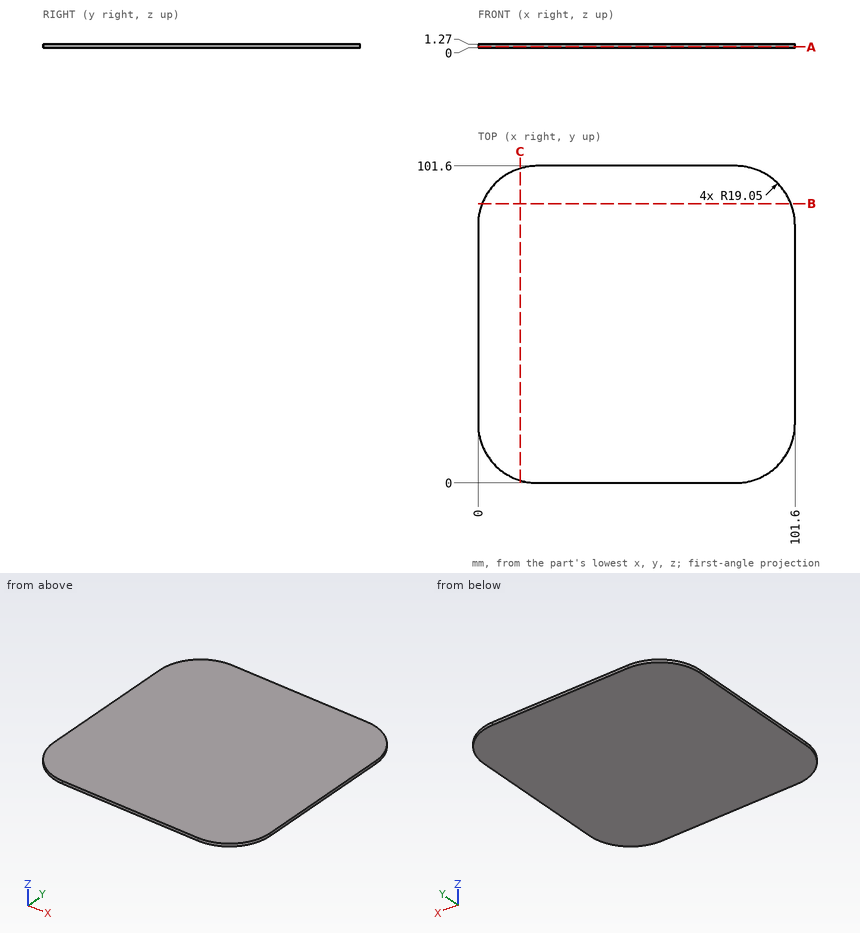
Part print with two shaded views. Sizes in mm from the minimum x, y, z corner. Round coordinates to 2 decimals unless told otherwise and drop trailing zeros. Loops run counter-clockwise (first coordinate to the right, second up) from the corner with the lowest first, then second, coordinate; pieces in that order, holes last. Notation, with made-up numbers: (26, 58) - (40, 58) arc R26 ccw to (40, 97) - close; hole circle Ø1 at (11.25, 32). An arc over 180 degrees is marked (long way). Put each result on its own line as item: value.
1. Slice it at B-B on y = 89.5. List the corners of the cut face in (x, z).
Geometry check:
outline: (1.31, 0) - (100.29, 0) - (100.29, 1.27) - (1.31, 1.27) - close
2. Slice it at A-A on z = 0.35. List the corners of the cut face in (x, y).
Geometry check:
outline: (0, 19.05) arc R19.05 ccw to (19.05, 0) - (82.55, 0) arc R19.05 ccw to (101.6, 19.05) - (101.6, 82.55) arc R19.05 ccw to (82.55, 101.6) - (19.05, 101.6) arc R19.05 ccw to (0, 82.55) - close
3. Slice it at C-C on x = 13.5. List the corners of the cut face in (y, z).
Geometry check:
outline: (0.83, 0) - (100.77, 0) - (100.77, 1.27) - (0.83, 1.27) - close
4. Wall check: line 1 (X direction, y = 96, z = 1); line 2 (Y direction, x = 84.5, z = 0.7); line 3 (X direction, y = 9.5, z = 1.15). Give the ranges that are in metal, low to high.
Geometry check:
line 1: 5.56 to 96.04
line 2: 0.1 to 101.5
line 3: 2.57 to 99.03
